Autodesk Inventor part; units mm, degrees
ref_plane "YZ Plane" through (0, 0, 0) normal (1, 0, 0) x (0, 1, 0)
ref_plane "XZ Plane" through (0, 0, 0) normal (0, 1, 0) x (-1, 0, 0)
ref_plane "XY Plane" through (0, 0, 0) normal (0, 0, 1) x (1, 0, 0)
sketch "Sketch1" plane through (0, 0, 0) normal (0, 1, 0) x (-1, 0, 0)
  line L0 (143.1818, 175) -> (143.1818, 172)
  line L1 (111.3636, 172) -> (111.3636, 175)
  line L2 (79.5455, 175) -> (79.5455, 172)
  line L3 (47.7273, 172) -> (47.7273, 175)
  line L4 (15.9091, 175) -> (15.9091, 172)
  line L5 (-15.9091, 172) -> (-15.9091, 175)
  line L6 (-47.7273, 175) -> (-47.7273, 172)
  line L7 (-79.5455, 172) -> (-79.5455, 175)
  line L8 (-111.3636, 175) -> (-111.3636, 172)
  line L9 (-143.1818, 172) -> (-143.1818, 175)
  line L10 (-175, 143.1818) -> (-172, 143.1818)
  line L11 (-172, 111.3636) -> (-175, 111.3636)
  line L12 (-175, 79.5455) -> (-172, 79.5455)
  line L13 (-172, 47.7273) -> (-175, 47.7273)
  line L14 (-175, 15.9091) -> (-172, 15.9091)
  line L15 (-172, -15.9091) -> (-175, -15.9091)
  line L16 (-172, -47.7273) -> (-175, -47.7273)
  line L17 (-175, -79.5455) -> (-172, -79.5455)
  line L18 (-172, -111.3636) -> (-175, -111.3636)
  line L19 (-175, -143.1818) -> (-172, -143.1818)
  line L20 (-143.1818, -175) -> (-143.1818, -172)
  line L21 (-111.3636, -172) -> (-111.3636, -175)
  line L22 (-79.5455, -175) -> (-79.5455, -172)
  line L23 (-47.7273, -172) -> (-47.7273, -175)
  line L24 (-15.9091, -172) -> (-15.9091, -175)
  line L25 (15.9091, -175) -> (15.9091, -172)
  line L26 (143.1818, -172) -> (143.1818, -175)
  line L27 (111.3636, -175) -> (111.3636, -172)
  line L28 (79.5455, -172) -> (79.5455, -175)
  line L29 (47.7273, -175) -> (47.7273, -172)
  line L30 (172, -143.1818) -> (175, -143.1818)
  line L31 (175, -111.3636) -> (172, -111.3636)
  line L32 (175, -79.5455) -> (172, -79.5455)
  line L33 (175, -15.9091) -> (172, -15.9091)
  line L34 (175, 15.9091) -> (172, 15.9091)
  line L35 (175, 143.1818) -> (172, 143.1818)
  line L36 (172, 111.3636) -> (175, 111.3636)
  line L37 (175, 79.5455) -> (172, 79.5455)
  line L38 (172, 47.7273) -> (175, 47.7273)
  line L39 (111.3636, -172) -> (143.1818, -172)
  line L40 (47.7273, -172) -> (79.5455, -172)
  line L41 (-15.9091, -172) -> (15.9091, -172)
  line L42 (172, -143.1818) -> (172, -111.3636)
  line L43 (172, -15.9091) -> (172, 15.9091)
  line L44 (172, 47.7273) -> (172, 79.5455)
  line L45 (172, 111.3636) -> (172, 143.1818)
  line L46 (143.1818, 172) -> (111.3636, 172)
  line L47 (79.5455, 172) -> (47.7273, 172)
  line L48 (15.9091, 172) -> (-15.9091, 172)
  line L49 (-47.7273, 172) -> (-79.5455, 172)
  line L50 (-111.3636, 172) -> (-143.1818, 172)
  line L51 (-172, 143.1818) -> (-172, 111.3636)
  line L52 (-172, 79.5455) -> (-172, 47.7273)
  line L53 (-172, 15.9091) -> (-172, -15.9091)
  line L54 (-175, 47.7273) -> (-175, 15.9091)
  line L55 (-175, 175) -> (-175, 143.1818)
  line L56 (-175, 111.3636) -> (-175, 79.5455)
  line L57 (-143.1818, -172) -> (-111.3636, -172)
  line L58 (-79.5455, -172) -> (-47.7273, -172)
  line L59 (-172, -47.7273) -> (-172, -79.5455)
  line L60 (-172, -111.3636) -> (-172, -143.1818)
  line L61 (-175, -15.9091) -> (-175, -47.7273)
  line L62 (-175, -79.5455) -> (-175, -111.3636)
  line L63 (-175, -143.1818) -> (-175, -175)
  line L64 (-175, -175) -> (-143.1818, -175)
  line L65 (-111.3636, -175) -> (-79.5455, -175)
  line L66 (-47.7273, -175) -> (-15.9091, -175)
  line L67 (15.9091, -175) -> (47.7273, -175)
  line L68 (79.5455, -175) -> (111.3636, -175)
  line L69 (143.1818, -175) -> (175, -175)
  line L70 (175, -175) -> (175, -143.1818)
  line L71 (175, 15.9091) -> (175, 47.7273)
  line L72 (175, 79.5455) -> (175, 111.3636)
  line L73 (175, 143.1818) -> (175, 175)
  line L74 (175, 175) -> (143.1818, 175)
  line L75 (111.3636, 175) -> (79.5455, 175)
  line L76 (47.7273, 175) -> (15.9091, 175)
  line L77 (-15.9091, 175) -> (-47.7273, 175)
  line L78 (-79.5455, 175) -> (-111.3636, 175)
  line L79 (-143.1818, 175) -> (-175, 175)
  line L80 (172, -79.5455) -> (172, -47.7273)
  line L81 (172, -47.7273) -> (175, -47.7273)
  line L82 (175, -111.3636) -> (175, -79.5455)
  line L83 (175, -47.7273) -> (175, -15.9091)
  point P0 (0, 0)
  dimension "d1" = 350
  dimension "d3" = 350
  dimension "d5" = 175
  dimension "d6" = 175
  dimension "d7" = 3
  dimension "d8" = 3
  dimension "d9" = 3
  dimension "d10" = 3
extrude "Extrusion1" add sketch "Sketch1" along normal blind 3
equation "\"d1\" = wt"
equation "\"d3\" = lt"
equation "\"d7\" = tt"
equation "\"d8\" = tt"
equation "\"d9\" = tt"
equation "\"d10\" = tt"
equation "\"d13\" = tt"
equation "\"wt\" = 350"
equation "\"tt\" = 3"
equation "\"tol\" = 0"
equation "\"tiroir\" = 25.4"
equation "\"nHoles\" = 101.6"
equation "\"shelfH\" = 35"
equation "\"d0\" = 0.5 * wt"
equation "\"d2\" = 0.5 * lt"
equation "\"lt\" = 350"
equation "\"d4\" = tt"
properties part number "base"
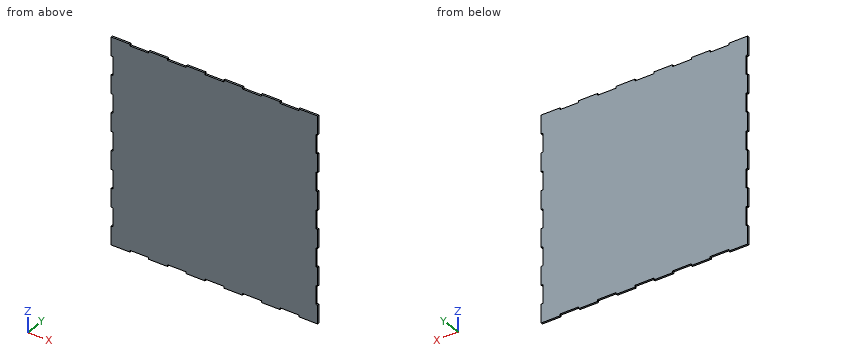
Here's how the part is built. I have some questions about the finished solid (model axes, mm). Round coordinates to 2 decimals unless told otherwise and drop trailing zeros. Order: outer loops, then holes, each group sorted by start corner. A loop starts at its lowest first (then second) coordinate and runs counter-clockwise, first axis right, second up. Notation, with made-up numbers: M 77.5,19 L 87.5,19 A25 ccw 87.5,41 Z; hole C 81.5,44 d10. An arc over 180 degrees is marked long. Use CSV: the item, a comma, the result in double quotes.
1) I want a section at B-B (x = 135.5). List the corners of the cut face in (y, z) for me, then the cut area to 3 significant figures.
Taken from the geometry:
outline,"M 0,-172 L 3,-172 L 3,172 L 0,172 Z"
area,"1,030 mm^2"
2) I'm going to push flat-ended pins straight in: P1, Ø1.5, axis at y = 1.5, z = -1, coming from the +X side; P2, Ø1, axis at y = 2, z = -116, coming from the -X side; P3, Ø1, axis at x = 53.5, y = 0.5, coming from the -Z side; P4, Ø8, axis at x = 81.5, z = -59.5, coming from the -Y side. Where does each tip first touch, or does it pass through?
Taken from the geometry:
P1,"x = 172"
P2,"x = -172"
P3,"z = -172"
P4,"y = 0"
3) I want a section at A-A (z = -70). List the corners of the cut face in (x, y) for me.
Taken from the geometry:
outline,"M -172,0 L 172,0 L 172,3 L -172,3 Z"
4) I need wall thicknesses on line 1 along Z through (x, y) = (-63.5, 1.4). Which ranges of the line are inside material? Lowest first, please. Write a range as [from, to].
Taken from the geometry:
line 1,"[-172, 172]"
